Check sheet for the modelled part. Datum: model origin and axes. Units: mm. Round coordinates to 2 decimals unless told otherwise and drop trailing zeros. Order: outer loops, then holes, each group sorted by start corner. A loop starts at its lowest first (then second) coordinate and runs counter-clockwise, first axis right, second up. Notation, with made-up numbers: (-38.75, 16.25) -> (0.25, 16.25) arc R26 ccw to (0.25, 48.25) -> close; hole circle Ø3 at (-4.75, 67.5). An arc over 180 degrees is marked (long way). Answer as CSV lines item,"result". Start each with the question number.
from build123d import *

# Parameters (mm, degrees)
BOSS_EXTRUDE1_DEPTH = 1.5875


with BuildPart() as part:
    # Sketch1 → Boss-Extrude1 (new, symmetric)
    with BuildSketch(Plane.XY):
        with BuildLine():
            Line((277.352525484, 130.514220253), (276.807932827, 136.840824305))
            Line((276.807932827, 136.840824305), (273.51809872, 136.557636124))
            Line((273.51809872, 136.557636124), (274.031797499, 130.589930281))
            ThreePointArc((274.031797499, 130.589930281), (230.30851429, 130.913472194), (186.59387592, 129.985805221))
            Line((186.59387592, 129.985805221), (186.349272737, 135.827805221))
            Line((186.349272737, 135.827805221), (183.050163268, 135.689672274))
            Line((183.050163268, 135.689672274), (183.294042864, 129.86495412))
            ThreePointArc((183.294042864, 129.86495412), (139.761460521, 127.601280315), (96.311168805, 124.096698424))
            ThreePointArc((96.311168805, 124.096698424), (95.971054745, 124.054032816), (95.631, 124.010897007))
            Line((95.631, 124.010897007), (95.631, 130.517973266))
            Line((95.631, 130.517973266), (92.329, 130.517973266))
            Line((92.329, 130.517973266), (92.329, 123.567152459))
            ThreePointArc((92.329, 123.567152459), (46.592607477, 112.602219611), (3.749926944, 93.197269774))
            Line((3.749926944, 93.197269774), (3.749926944, 100.055269774))
            Line((3.749926944, 100.055269774), (0, 100.055269774))
            Line((0, 100.055269774), (0, 101.6))
            ThreePointArc((0, 101.6), (1.157792804, 105.775489723), (4.300521626, 108.758517405))
            ThreePointArc((4.300521626, 108.758517405), (48.266347056, 127.216011607), (94.854415026, 137.375973266))
            ThreePointArc((94.854415026, 137.375973266), (326.208122032, 141.94293007), (555.638244479, 111.822940798))
            Line((555.638244479, 111.822940798), (558.229469453, 97.627349478))
            ThreePointArc((558.229469453, 97.627349478), (418.553478483, 120.58290755), (277.352525484, 130.514220253))
        make_face()
    extrude(amount=BOSS_EXTRUDE1_DEPTH, both=True)


solid = part.part
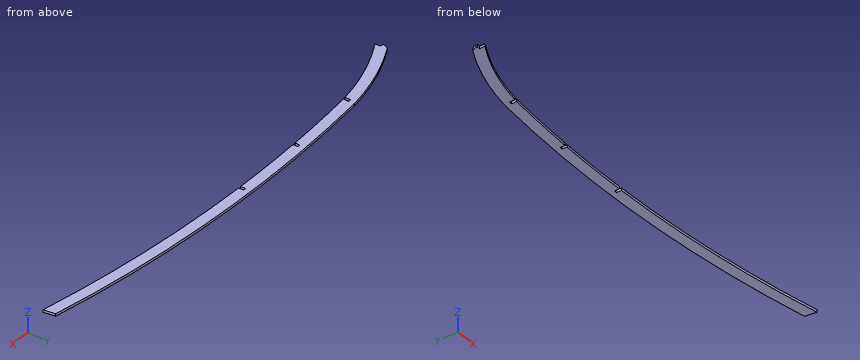
1) Material ranges on line 1 along Y through (x, z) = (120.5, -0.3); line 2 along Y through (x, z) = (173.5, 0); line 3 along X through (y, z) = (96, -1.1), recorded low to high.
2) Section check C-C on x = 243. Record the cut outline in (y, z), then the cut area to 3 significant figures.
3) Section check D-D on x = 463. Record the cut outline in (y, z), then the cut area to 3 significant figures.
4) Section check B-B on z = 0.65. Record the cut outline in (x, y).
5) Depth check by flat-ended pin: pin 1 Ø1 at (y, z) = (110, 0) entering from -X; pin 2 Ø1 at (x, z) = (94.5, -0.5) entering from -Y; pin 3 Ø5 at (x, y) = (101, 119.5) entering from +Z. Enter the tip coordinate at first touch or a pass-through.
Solutions:
1,line 1,"y = 126.2 to 139.6"
1,line 2,"y = 129.46 to 142.83"
1,line 3,"x = 3.75 to 8.78"
2,outline,"(130.95, -1.59) -> (144.31, -1.59) -> (144.31, 1.59) -> (130.95, 1.59) -> close"
2,area,"42.4 mm^2"
3,outline,"(114.72, -1.59) -> (128.22, -1.59) -> (128.22, 1.59) -> (114.72, 1.59) -> close"
3,area,"42.9 mm^2"
4,outline,"(0, 100.06) -> (3.75, 100.06) -> (3.75, 93.2) arc R247.92 cw to (92.33, 123.57) -> (92.33, 130.52) -> (95.63, 130.52) -> (95.63, 124.01) arc R247.92 cw to (96.31, 124.1) arc R1527.95 cw to (183.29, 129.86) -> (183.05, 135.69) -> (186.35, 135.83) -> (186.59, 129.99) arc R1527.95 cw to (274.03, 130.59) -> (273.52, 136.56) -> (276.81, 136.84) -> (277.35, 130.51) arc R1527.95 cw to (558.23, 97.63) -> (555.64, 111.82) arc R1541.31 ccw to (94.85, 137.38) arc R261.28 ccw to (4.3, 108.76) arc R8.11 ccw to (0, 101.6) -> close"
5,pin 1,"stops at x = 5.7"
5,pin 2,"stops at y = 130.52"
5,pin 3,"passes through"
